Model file for the job. Use its own axes, mm. A direction names the side the tool comes from. Round coordinates to 2 decimals unless told otherwise and drop trailing zeros. Loops run counter-clockwise (first coordinate to the right, second up) from the corner with the lowest first, then second, coordinate; pieces in that order, holes last. Notation, with made-up numbers: M -6.5,58 L 49.5,58 A11 cw 49.5,78 Z; hole C -13,76.5 d9. An arc over 180 degrees is marked long. Use a Markdown table: item, result. Add a question column.
Item 1: Wall check: L1, parallel to Z at x = -62.5, y = 16.25; L2, parallel to X at y = 17.1, z = -19; L3, parallel to Z at x = -104.5, y = 1.75. Give the ranges that are in metal, low to high. Write a range as from..to.
Item 2: Tool access for faces 1 (the flat face through (-122.5, 7, -19)), 2 (the cylindrical face through (-74.6, 1.52, 11.14)), 3 (the flat face through (-64, 18, -17)), 4 (the flat face through (-62, 14, 17)), 5 (the cylindrical face through (-119.641, 1.479, -14.297)): list every direction of +Z, -Z, +X, -X, +Y, -Y with a clear straight run to the whole face (end or side of a thin tool).
Item 3: Two-plate mould, pull along Z, no slides. Class faces 6 (the cylindrical face through (-107.094, 0.74, -10.411)), 7 (the flat face through (-68, 11, -12)), 8 (the cylindrical face through (-58.4, 16.03, -21.64)), 9 (the flat face through (-118.5, 11, -19)): +Z half, -Z half, draft (parallel to the pull), parting line (faces both ways), or undercut.
Item 4: Saw through at A-A on y = 17. Write the cut outline in (x, z), then the cut area to 3 significant figures.
Item 5: Pin check, flat tips, straight feed: P1, Ø5, axis at x = -127.5, z = -19, coming from the -Y side; P2, Ø4, axis at x = -84.39, z = 10.61, coming from the +Y side; P3, Ø3, axis at y = 6, z = -18, coming from the +X side; P4, Ø4, axis at x = -105.61, z = -10.61, coming from the -Y side. Stop position of each tip, or through.
Item 6: Saw through at D-D on y = 4. Write the cut outline in (x, z).
Item 7: Saw through at B-B on x = -127.5. Write the cut outline in (y, z).
Item 8: Saw through at C-C on z = -4. Write the cut outline in (x, y).
```python
from build123d import *

# Parameters (mm, degrees)
SKETCH_1_W          = 75
SKETCH_1_H          = 45
EXTRUDE_1_DEPTH     = 18
SKETCH_2_W          = 10
SKETCH_2_H          = 45
CUT_EXTRUDE_1_DEPTH = 14
SKETCH_3_W          = 47
SKETCH_3_H          = 45
CUT_EXTRUDE_2_DEPTH = 15
SKETCH_4_R          = 1.5
SKETCH_4_R_2        = 7.5
CUT_EXTRUDE_3_DEPTH = 48.291648311
SKETCH_5_W          = 14
SKETCH_5_H          = 38
CUT_EXTRUDE_4_DEPTH = 48.291648311
FILLET_1_R          = 30
CHAMFER_1_SIZE      = 1.5
SKETCH_8_W          = 36
SKETCH_8_H          = 24
CUT_EXTRUDE_6_DEPTH = 48.291648311
FILLET_2_R          = 3
SKETCH_9_R          = 1.5
CUT_EXTRUDE_7_DEPTH = 46.918405896
FILLET_3_R          = 3
FILLET_4_R          = 4
SKETCH_10_W         = 113.481705681
SKETCH_10_H         = 81.455057911
CUT_EXTRUDE_9_DEPTH = 136.596828871


with BuildPart() as part:
    # 草图1 → 凸台-拉伸1 (new body)
    with BuildSketch(Plane(origin=(0, 0, 0), x_dir=(1, 0, 0), z_dir=(0, 1, 0))):
        Rectangle(SKETCH_1_W, SKETCH_1_H)
    extrude(amount=EXTRUDE_1_DEPTH)

    # 草图2 → 切除-拉伸1 (cut)
    with BuildSketch(Plane.XZ):
        with Locations((-32.5, 0)):
            Rectangle(SKETCH_2_W, SKETCH_2_H)
        with Locations((32.5, 0)):
            Rectangle(SKETCH_2_W, SKETCH_2_H)
    extrude(amount=-CUT_EXTRUDE_1_DEPTH, mode=Mode.SUBTRACT)

    # 草图3 → 切除-拉伸2 (cut)
    with BuildSketch(Plane(origin=(0, 18, 0), x_dir=(1, 0, 0), z_dir=(0, 1, 0))):
        Rectangle(SKETCH_3_W, SKETCH_3_H)
    extrude(amount=-CUT_EXTRUDE_2_DEPTH, mode=Mode.SUBTRACT)

    # 草图4 → 切除-拉伸3 (cut, through all)
    with BuildSketch(Plane.XZ):
        with Locations(Location((10.606601718, 10.606601718, 0), (0, 0, 270))):
            Circle(SKETCH_4_R)
        with Locations(Location((10.606601718, -10.606601718, 0), (0, 0, 270))):
            Circle(SKETCH_4_R)
        with Locations(Location((-10.606601718, -10.606601718, 0), (0, 0, 270))):
            Circle(SKETCH_4_R)
        with Locations(Location((-10.606601718, 10.606601718, 0), (0, 0, 270))):
            Circle(SKETCH_4_R)
        with Locations(Location((0, 0, 0), (0, 0, 270))):
            Circle(SKETCH_4_R_2)
    extrude(amount=-CUT_EXTRUDE_3_DEPTH, mode=Mode.SUBTRACT)

    # 草图5 → 切除-拉伸4 (cut, through all)
    with BuildSketch(Plane(origin=(0, 18, 0), x_dir=(1, 0, 0), z_dir=(0, 1, 0))):
        with Locations((30.5, -3.5)):
            Rectangle(SKETCH_5_W, SKETCH_5_H)
    extrude(amount=-CUT_EXTRUDE_4_DEPTH, mode=Mode.SUBTRACT)

    # 圆角1
    fillet_1_edges = [part.edges().sort_by_distance(p)[0] for p in [
        (23.5, 1.5, 22.5),
    ]]
    fillet(fillet_1_edges, radius=FILLET_1_R)

    # 倒角1
    chamfer_1_edges = [part.edges().sort_by_distance(p)[0] for p in [
        (-10.606601718, 3, 12.106601718),
        (-10.606601718, 3, -9.106601718),
        (10.606601718, 3, -9.106601718),
        (10.606601718, 3, 12.106601718),
    ]]
    chamfer(chamfer_1_edges, length=CHAMFER_1_SIZE)

    # 草图8 → 切除-拉伸6 (cut, through all)
    with BuildSketch(Plane.XZ):
        with Locations((-37.5, 0)):
            Rectangle(SKETCH_8_W, SKETCH_8_H)
    extrude(amount=-CUT_EXTRUDE_6_DEPTH, mode=Mode.SUBTRACT)

    # 圆角2
    fillet_2_edges = [part.edges().sort_by_distance(p)[0] for p in [
        (-19.5, 1.5, 12),
        (-19.5, 1.5, -12),
    ]]
    fillet(fillet_2_edges, radius=FILLET_2_R)

    # 草图9 → 切除-拉伸7 (cut, through all)
    with BuildSketch(Plane.XZ.offset(-14)):
        with Locations(Location((32.5, -19, 0), (0, 0, 270))):
            Circle(SKETCH_9_R)
        with Locations(Location((-32.5, -19, 0), (0, 0, 270))):
            Circle(SKETCH_9_R)
        with Locations(Location((-32.5, 19, 0), (0, 0, 270))):
            Circle(SKETCH_9_R)
    extrude(amount=-CUT_EXTRUDE_7_DEPTH, mode=Mode.SUBTRACT)

    # 圆角3
    fillet_3_edges = [part.edges().sort_by_distance(p)[0] for p in [
        (-37.5, 16, 12),
        (-37.5, 16, -12),
        (-37.5, 16, 22.5),
        (-37.5, 16, -22.5),
        (37.5, 16, -22.5),
        (37.5, 16, -15.5),
    ]]
    fillet(fillet_3_edges, radius=FILLET_3_R)

    # 圆角4
    fillet_4_edges = [part.edges().sort_by_distance(p)[0] for p in [
        (23.5, 1.5, -15.5),
    ]]
    fillet(fillet_4_edges, radius=FILLET_4_R - 0.0001)  # a hair under: the kernel refuses the full size


with BuildPart() as body_2:
    # 镜向1: mirrored copy
    add(part.part.mirror(Plane.ZY.offset(47.5)))


with BuildPart() as part_1:
    add(part.part)

    # 草图10 → 切除-拉伸9 (cut, through all)
    with BuildSketch(Plane.XZ):
        with Locations((9.796228236, -0.64793796)):
            Rectangle(SKETCH_10_W, SKETCH_10_H)
    extrude(amount=-CUT_EXTRUDE_9_DEPTH, mode=Mode.SUBTRACT)


solid = body_2.part
```
Entries:
| question | item | result |
|---|---|---|
| 1 | L1 | -22.5..-20.5, -17.5..-12, 12..17.5, 20.5..22.5 |
| 1 | L2 | -132.5..-129, -126..-118.5, -71.5..-64, -61..-57.5 |
| 1 | L3 | -22.5..-11.96, -9.25..9.25, 11.96..17.88 |
| 2 | face 1 | +Z, -Z, -X, -Y |
| 2 | face 2 | +X, +Y, -Y |
| 2 | face 3 | +Z, -Z, +X, -X, +Y |
| 2 | face 4 | +Z, -Z, +X, -Y |
| 2 | face 5 | +Z, -X, +Y, -Y |
| 3 | face 6 | undercut |
| 3 | face 7 | undercut |
| 3 | face 8 | -Z half |
| 3 | face 9 | draft |
| 4 | outline | M -132.5,-19.5 A3 ccw -129.5,-22.5 L -118.5,-22.5 L -118.5,-15.5 L -129.5,-15.5 A3 ccw -132.5,-18.5 Z; M -71.5,-22.5 L -60.5,-22.5 A3 ccw -57.5,-19.5 L -57.5,-15 A3 ccw -60.5,-12 L -71.5,-12 Z; M -71.5,12 L -60.5,12 A3 ccw -57.5,15 L -57.5,19.5 A3 ccw -60.5,22.5 L -71.5,22.5 Z; hole C -127.5,-19 d3; hole C -62.5,-19 d3; hole C -62.5,19 d3 |
| 4 | area | 359 mm2 |
| 5 | P1 | y = 14 |
| 5 | P2 | y = 2 |
| 5 | P3 | x = -67.5 |
| 5 | P4 | y = 0 |
| 6 | outline | M -122.5,-22.5 L -118.5,-22.5 L -118.5,-15.5 L -122.5,-15.5 Z; M -71.5,-22.5 L -67.5,-22.5 L -67.5,-12 L -71.5,-12 Z; M -71.5,12 L -67.5,12 L -67.5,22.5 L -71.5,22.5 Z |
| 7 | outline | M 14,-22.5 L 18,-22.5 L 18,-20.5 L 14,-20.5 Z; M 14,-17.5 L 18,-17.5 L 18,-15.5 L 14,-15.5 Z |
| 8 | outline | M -118.3,0 L -101.34,0 L -101.34,3 L -118.3,3 Z; M -88.66,0 L -75.5,0 L -75.5,3 L -88.66,3 Z |
